from build123d import *

# Parameters (mm, degrees)
F0_R        = 18.3
F1_DEPTH    = 110
F0_R_2      = 24
F0_R_3      = 19.5
F2_DEPTH    = 30
F3_S5_R     = 18.3
F3_T6_DEPTH = 36
F4_SIZE2    = 17
F4_SIZE     = 15
F5_R        = 10
F6_T        = -0.8
F7_DEPTH    = 25


# Not quite as in the source:
# - a fillet or chamfer that OpenCascade refuses, or shapes differently, is made with other operations: its cross-section is extruded or revolved along the edge and cut away or added


with BuildPart() as f1:
    # F0 (on Top) → F1 (new body)
    with BuildSketch(Plane.XY):
        Circle(F0_R)
    extrude(amount=F1_DEPTH)

    # F0 (on Top) → F2 (join)
    with BuildSketch(Plane.XY):
        Circle(F0_R_2)
        Circle(F0_R_3, mode=Mode.SUBTRACT)
        Circle(F0_R_3)
        Circle(F0_R, mode=Mode.SUBTRACT)
    extrude(amount=F2_DEPTH)

    # F3: chamfer of 7 x 14 on 1 edges, made by hand


with BuildPart() as f3_tool2:
    # F3_s3 → F3_t4 (revolve)
    with BuildSketch(Plane.XZ):
        Polygon((17, 30), (24, 16), (24, 30), align=None)
    revolve(axis=Axis((0, 0, 30), (0, 0, 1)))

    # F3_s5 → F3_t6 (cut, symmetric)
    with BuildSketch(Plane.XY.offset(23)):
        Circle(F3_S5_R)
    extrude(amount=F3_T6_DEPTH, both=True, mode=Mode.SUBTRACT)


with BuildPart() as f1_1:
    add(f1.part)

    # F3_t1: cut F3_tool2
    add(f3_tool2.part, mode=Mode.SUBTRACT)

    # F4
    f4_edges = [f1_1.edges().sort_by_distance(p)[0] for p in [
        (-18.3, 0, 110),
    ]]
    f4_side = f1_1.faces().sort_by_distance((0, 0, 110))[0]
    chamfer(f4_edges, length=F4_SIZE, length2=F4_SIZE2, reference=f4_side)

    # F5
    f5_edges = [f1_1.edges().sort_by_distance(p)[0] for p in [
        (-18.3, 0, 93),
        (-18.3, 0, 30),
        (-18.3, 0, 27.4),
        (-24, 0, 16),
    ]]
    fillet(f5_edges, radius=F5_R)

    # F6
    f6_openings = [f1_1.faces().sort_by_distance(p)[0] for p in [
        (0, 0, 0),
    ]]
    offset(amount=F6_T, openings=f6_openings)

    # F7 (cut): a face of the model
    f7_faces = [f1_1.faces().sort_by_distance(p)[0] for p in [
        (0, 0, 110),
    ]]
    extrude(f7_faces, amount=-F7_DEPTH, mode=Mode.SUBTRACT)


solid = f1_1.part
Can you work these out from the model? Positions are in its coordinate system, mm. A direction names the side the tool comes from. Coordinates: 2 decimals unless noted, no trailing zeros. Write each loop counter-clockwise with the first axis right and the second up, starting at its lowest first coordinate (ties: lowest second). Pieces come first, ordered by that corner, then holes. Notation, with made-up numbers: (-26.5, 51) - (14.5, 51) arc R15 cw to (14.5, 74) - close; hole circle Ø4 at (8, 58). An arc over 180 degrees is marked (long way). Return JSON: item names as keys, results as strings. Group by question number.
Item 1: If we section it at A-A (z = 34.5): Write out the boundary of the cut face in (x, y), then the cut area to 3 significant figures.
Item 2: We'd pull the mould along Y, two halves only. Please class faces 1 (the face through (8.075, -15.526, 59.074)), 2 (the face through (-12.6, 19.7, 0)), 3 (the face through (5.05, -2.1, 107.54)): pulls with the +Y half, pulls with the -Y half, needs draft (parallel to the pull), parting line crosses it, or undercut.
Item 3: If we section it at B-B (z = 101.5): Write out the boundary of the cut face in (x, y).
Item 4: Which directions (+Z, -Z, +X, -X, +Y, -Y) give clear straight access to the entire face, cutting with the end or side of a thin tool? Please do faces 4 (the face through (-23.178, 1.02, 6.724)), 5 (the face through (9.04, -17.37, 24.84)).
Item 5: I'm going to push flat-ended pins straight in: pin 1 Ø1.5 at (x, z) = (-12, 94) entering from -Y; pin 2 Ø4 at (x, y) = (0, 0) entering from +Z; pin 3 Ø6 at (y, z) = (-6.5, 30.5) entering from -X; pin 4 Ø5 at (x, y) = (10.5, -6) entering from -Z. Where does each tip first touch, or does it pass through?
Item 6: Please list where these lines run through material, in increasing order: probe 1 along Y at (x, z) = (0, 8); probe 2 along Y at (x, z) = (0, 109.3).
Return value:
{
 "1": {"outline": "circle Ø36.6 at (0, 0); hole circle Ø35 at (0, 0)", "area": "90.0 mm^2"},
 "2": {"face 1": "undercut", "face 2": "needs draft", "face 3": "parting line crosses it"},
 "3": {"outline": "circle Ø21.6 at (0, 0); hole circle Ø19.47 at (0, 0)"},
 "4": {"face 4": "-Z", "face 5": "+Z"},
 "5": {"pin 1": "stops at y = -13.03", "pin 2": "passes through", "pin 3": "stops at x = -17.96", "pin 4": "stops at z = 95.99"},
 "6": {"probe 1": "y = -24 to -23.2, 23.2 to 24", "probe 2": "y = -3.92 to -3.3, 3.3 to 3.92"}
}
